```python
from build123d import *

# Parameters (mm, degrees)
F0_W     = 21
F0_H     = 25
F1_DEPTH = 0.5
F3_DEPTH = 25
F4_W     = 4.5
F4_H     = 5
F5_DEPTH = 25


with BuildPart() as f1:
    # F0 (on Front) → F1 (new body)
    with BuildSketch(Plane.XZ):
        with Locations((2.391892, 2.5)):
            Rectangle(F0_W, F0_H)
    extrude(amount=F1_DEPTH)

    # F2 (on face) → F3 (cut)
    with BuildSketch(Plane.XZ.offset(0.5)):
        with BuildLine():
            ThreePointArc((-5.358108, -6), (-3.10796, -8.25), (-0.858108, -5.999706))
            Line((-0.858108, -5.999706), (-0.858108, 2.000294))
            ThreePointArc((-0.858108, 2.000294), (-3.108255, 4.25), (-5.358108, 2))
            Line((-5.358108, 2), (-5.358108, -6))
        make_face()
        with BuildLine():
            Line((5.641892, 2.000294), (5.641892, -5.999706))
            ThreePointArc((5.641892, -5.999706), (7.891745, -8.25), (10.141892, -6))
            Line((10.141892, -6), (10.141892, 2))
            ThreePointArc((10.141892, 2), (7.89204, 4.25), (5.641892, 2.000294))
        make_face()
    extrude(amount=-F3_DEPTH, mode=Mode.SUBTRACT)

    # F4 (on face) → F5 (cut)
    with BuildSketch(Plane.XZ.offset(0.5)):
        with Locations((2.391892, 9)):
            Rectangle(F4_W, F4_H)
        with BuildLine():
            Line((0.141892, 11.5), (4.641892, 11.5))
            ThreePointArc((4.641892, 11.5), (2.391892, 13.75), (0.141892, 11.5))
        make_face()
        with BuildLine():
            ThreePointArc((0.141892, 6.5), (2.391892, 4.25), (4.641892, 6.5))
            Line((4.641892, 6.5), (0.141892, 6.5))
        make_face()
    extrude(amount=-F5_DEPTH, mode=Mode.SUBTRACT)


solid = f1.part
```
Input: part model. Units: mm. Frame: model coordinates. A direction names the side the tool comes from. Give positions to 0.01 mm unless a question says otherwise; leave off trailing zeros. Order: outer loops, then holes, each group sorted by start corner. A loop starts at its lowest first (then second) coordinate and runs counter-clockwise, first axis right, second up. Notation, with made-up numbers: M -23.75,44.25 L -16.75,44.25 A21 cw -16.75,80.25 Z; hole C 44,24.5 d5. An arc over 180 degrees is marked long. One line per question, with ' | ' between items. Start each with the question number.
1. Section query B-B (y = -0.4). Return the cut outline in (x, z), and give its area (3 significant figures).
2. Pull-direction query (Z, two-part tool) for faces 1 (the face through (2, 0, 3)), 2 (the face through (7.94, -0.25, 4.25)); classes: released by +Z, released by -Z, zero draft, split by the parting line, or undercut.
3. Section query D-D (z = -5). Return the cut outline in (x, y), and give its area (3 significant figures).
4. Section query C-C (x = 4.25). Return the cut outline in (y, z), and give its area (3 significant figures).
5. Section query A-A (z = 9.5). Return the cut outline in (x, y), and give its area (3 significant figures).
6. Material intervals for probe 1 along X at (y, z) = (-0.15, -5.5); probe 2 along X at (y, z) = (-0.2, 11.25); probe 3 along Z at (x, y) = (2.5, -0.05), sorted ascending. Write a range as [from, to].
7. Access query for faces 3 (the face through (2, -0.5, 3)), 4 (the face through (7.84, -0.25, -8.25)). Directions: +Z, -Z, +X, -X, +Y, -Y. A direction counts if a zero-diameter tool reaches every point of the face in a straight line with its end or side. Return the directions, or none.
Here are the results:
1) outline: M -8.11,-10 L 12.89,-10 L 12.89,15 L -8.11,15 Z; hole M -5.36,-6 A2.25 ccw -0.86,-6 L -0.86,2 A2.25 ccw -5.36,2 Z; hole M 0.14,6.5 A2.25 ccw 4.64,6.5 L 4.64,11.5 A2.25 ccw 0.14,11.5 Z; hole M 5.64,-6 A2.25 ccw 10.14,-6 L 10.14,2 A2.25 ccw 5.64,2 Z | area: 383 mm²
2) face 1: zero draft | face 2: undercut
3) outline: M -8.11,-0.5 L -5.36,-0.5 L -5.36,0 L -8.11,0 Z; M -0.86,-0.5 L 5.64,-0.5 L 5.64,0 L -0.86,0 Z; M 10.14,-0.5 L 12.89,-0.5 L 12.89,0 L 10.14,0 Z | area: 6.00 mm²
4) outline: M -0.5,-10 L 0,-10 L 0,5.23 L -0.5,5.23 Z; M -0.5,12.77 L 0,12.77 L 0,15 L -0.5,15 Z | area: 8.73 mm²
5) outline: M -8.11,-0.5 L 0.14,-0.5 L 0.14,0 L -8.11,0 Z; M 4.64,-0.5 L 12.89,-0.5 L 12.89,0 L 4.64,0 Z | area: 8.25 mm²
6) probe 1: [-8.11, -5.36], [-0.86, 5.64], [10.14, 12.89] | probe 2: [-8.11, 0.14], [4.64, 12.89] | probe 3: [-10, 4.25], [13.75, 15]
7) face 3: +Z, -Z, +X, -X, -Y | face 4: +Y, -Y
